For this review, use the dimensioned drawing (mm, ordinates from the lowest corner) and the shaded views. A direction names the side the tool comes from. Coordinates: 2 decimals unless noted, no trailing zeros. Loops run counter-clockwise (first coordinate to the right, second up) from the corner with the lowest first, then second, coordinate; pieces in that order, holes last. Notation, with made-up numbers: (16.5, -34.75) - (32.5, -34.75) arc R12 cw to (32.5, -18.75) - close; hole circle Ø8 at (3, 60). An arc over 180 degrees is marked (long way). One line per item, written item: value. Start each with the question number.
1. Mouldability with a two-part tool opening along Y and no side actions: class the marked faces 1, 2 and 3 as +Y half, -Y half, draft (parallel to the pull), parting line (faces both ways), or undercut.
2. For the marked faces 4 and 5, list the 3-axis set-ups (+Z, -Z, +X, -X, +Y, -Y) from which the entire face can be reached by the end or side of a thin tool; tool diameter is ignored.
3. We need section C-C, the plane z = 17. Give the boundary of the cut face in (x, y), then the cut area to 3 significant figures.
4. To check wall thickness, follow line 1 (Y direction, x = 9.9, z = 3); line 2 (X direction, y = 10.25, z = 2.5); line 3 (Z direction, x = 11, y = 12). State the ranges of each line that lie inside material, in increasing order.
5. We need section A-A, the plane x = 9.9. Give the boundary of the cut face in (y, z), then the cut area to 3 significant figures.
6. We need section D-D, the plane x = 5.5. Give the boundary of the cut face in (y, z).
7. Insertion check: P1, Ø2, axis at y = 15.5, z = 5.5, coming from the -X side; P2, Ø4.5, axis at x = 12.5, y = 13, coming from the -Z side; P3, Ø8, axis at x = 12.5, z = 35.5, coming from the +Y side; P4, Ø3, axis at y = 4, z = 21.5, coming from the +X side. Each pin has a flat end and moves straight along its axis. Give the tip position at first contact, or say it passes through.
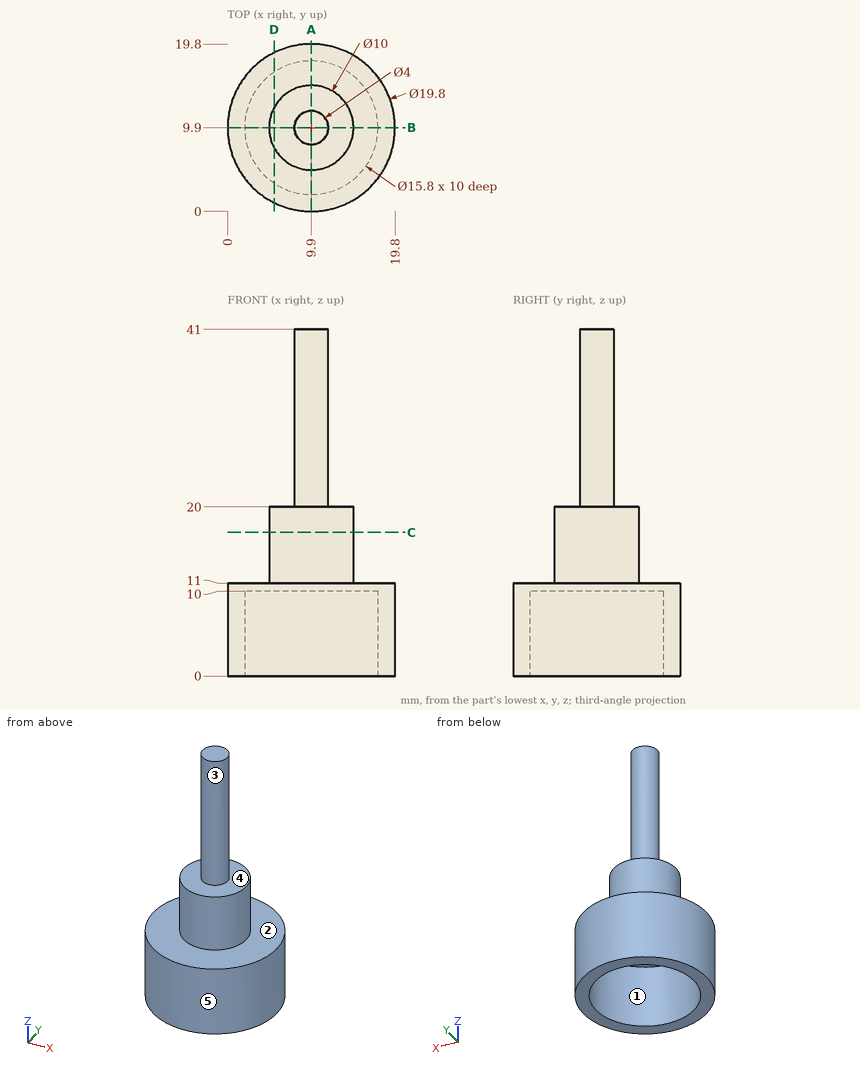
Findings below:
1. face 1: undercut
1. face 2: draft
1. face 3: parting line
2. face 4: +Z
2. face 5: +Z, -Z
3. outline: circle Ø10 at (9.9, 9.9)
3. area: 78.5 mm2
4. line 1: 0 to 2, 17.8 to 19.8
4. line 2: 0.01 to 2.01, 17.79 to 19.79
4. line 3: 10 to 20
5. outline: (0, 0) - (2, 0) - (2, 10) - (17.8, 10) - (17.8, 0) - (19.8, 0) - (19.8, 11) - (14.9, 11) - (14.9, 20) - (11.9, 20) - (11.9, 41) - (7.9, 41) - (7.9, 20) - (4.9, 20) - (4.9, 11) - (0, 11) - close
5. area: 234 mm2
6. outline: (1.03, 0) - (3.34, 0) - (3.34, 10) - (16.46, 10) - (16.46, 0) - (18.77, 0) - (18.77, 11) - (12.27, 11) - (12.27, 20) - (7.53, 20) - (7.53, 11) - (1.03, 11) - close
7. P1: x = 1.13
7. P2: z = 10
7. P3: y = 11.9
7. P4: through
